Autodesk Inventor part; units mm, degrees
ref_plane "YZ Plane" through (0, 0, 0) normal (1, 0, 0) x (0, 1, 0)
ref_plane "XZ Plane" through (0, 0, 0) normal (0, 1, 0) x (-1, 0, 0)
ref_plane "XY Plane" through (0, 0, 0) normal (0, 0, 1) x (1, 0, 0)
sketch "Sketch2" plane through (0, 0, 0) normal (0, 1, 0) x (-1, 0, 0)
  circle A0 centre (0, 0) radius 3.1
  circle A1 centre (0, 0) radius 12
  circle A2 centre (8, 0) radius 1.23
  circle A3 centre (4, 6.9282) radius 1.23
  circle A4 centre (-4, 6.9282) radius 1.23
  circle A5 centre (-8, 0) radius 1.23
  circle A6 centre (-4, -6.9282) radius 1.23
  circle A7 centre (4, -6.9282) radius 1.23
  dimension "d12" = 6.2
  dimension "d14" = 24
  dimension "d15" = 2.46
  dimension "d16" = 0
  dimension "d17" = 8
  dimension "d20" = 360
extrude "Extrusion2" add sketch "Sketch2" along normal blind 26.68
properties part number "smallSprocketHolder" material "ABS Plastic"
Work out the finished part from the listing and answer in its coordinate system (mm). Give positions to 0.01 mm unless a question says otherwise; leave off trailing zeros. Loops run counter-clockwise (first coordinate to the right, second up) from the corner with the lowest first, then second, coordinate; pieces in that order, holes last. Notation, with made-up numbers: (-13.5, 51) -> (33.5, 51) arc R19 ccw to (33.5, 85) -> close; hole circle Ø9 at (34, 8). An arc over 180 degrees is marked (long way). Use a Markdown table: item, result. Add a question column.
1) The part is cut by section D-D, the plane z = 4.25. Determine the outline of the cut face in (x, y).
2) The part is cut by section A-A, the plane x = 0. Determine the outline of the cut face in (y, z).
3) For a pull along Z with two mould halves and no side action, classify faces 1 (the flat face through (-2.5, 26.68, -2.5)), 2 (the cylindrical face through (4.16, 13.153, -8.148)), 3 (the cylindrical face through (11.99, 13.15, -0.53)), 4 (the cylindrical face through (-3.093, 13.153, -7.759)) as +Z half, -Z half, draft (parallel to the pull), parting line (faces both ways), or undercut.
4) The part is cut by section C-C, the plane y = 9.75. Determine the outline of the cut face in (x, z), plus the area to 3 significant figures.
5) The part is cut by section B-B, the plane x = -4. Determine the outline of the cut face in (y, z), plus the area to 3 significant figures.
6) Consider line 1 along Z through (x, y) = (-4, 16.75); line 2 along Z through (x, y) = (-4.5, 5); line 3 along X through (y, z) = (14, -7.25). Determine where each line is inside the solid, lowest interval first.
7) Each of these flat-tipped pins is pushed along its axis until it touches: P1, Ø5.5, axis at x = 0, z = 0, coming from the -Y side; P2, Ø10, axis at y = 11, z = -8, coming from the +X side; P3, Ø2, axis at y = 16.5, z = -6, coming from the +X side; P4, Ø3, axis at x = -8, y = 3.5, coming from the +Z side. Where does it stop, or does it pass through?
Reported:
| question | item | result |
|---|---|---|
| 1 | outline | (-11.22, 0) -> (11.22, 0) -> (11.22, 26.68) -> (-11.22, 26.68) -> close |
| 2 | outline | (0, -12) -> (26.68, -12) -> (26.68, -3.1) -> (0, -3.1) -> close; (0, 3.1) -> (26.68, 3.1) -> (26.68, 12) -> (0, 12) -> close |
| 3 | face 1 | draft |
| 3 | face 2 | undercut |
| 3 | face 3 | parting line |
| 3 | face 4 | undercut |
| 4 | outline | circle Ø24 at (0, 0); hole circle Ø2.46 at (-8, 0); hole circle Ø2.46 at (-4, -6.93); hole circle Ø2.46 at (-4, 6.93); hole circle Ø6.2 at (0, 0); hole circle Ø2.46 at (4, -6.93); hole circle Ø2.46 at (4, 6.93); hole circle Ø2.46 at (8, 0) |
| 4 | area | 394 mm^2 |
| 5 | outline | (0, -11.31) -> (26.68, -11.31) -> (26.68, -8.16) -> (0, -8.16) -> close; (0, -5.7) -> (26.68, -5.7) -> (26.68, 5.7) -> (0, 5.7) -> close; (0, 8.16) -> (26.68, 8.16) -> (26.68, 11.31) -> (0, 11.31) -> close |
| 5 | area | 472 mm^2 |
| 6 | line 1 | z = -11.31 to -8.16, -5.7 to 5.7, 8.16 to 11.31 |
| 6 | line 2 | z = -11.12 to -8.05, -5.8 to 5.8, 8.05 to 11.12 |
| 6 | line 3 | x = -9.56 to -5.19, -2.81 to 2.81, 5.19 to 9.56 |
| 7 | P1 | passes through |
| 7 | P2 | stops at x = 11.62 |
| 7 | P3 | stops at x = 10.91 |
| 7 | P4 | stops at z = 10.09 |
